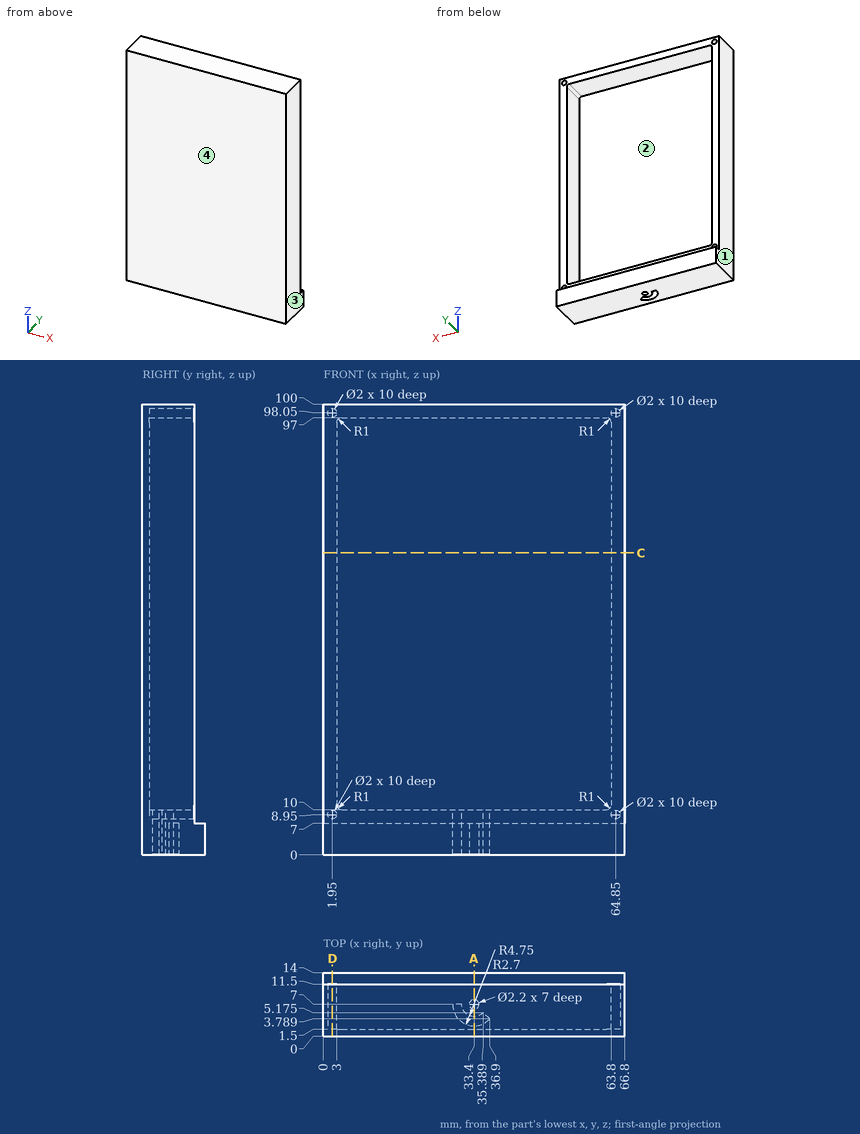
The figure shows three views and two pictorial views of one solid part (mm, origin at its lowest corner). Answer the questions. Give positions to 0.01 mm unless a question says otherwise; leave off trailing zeros. Order: outer loops, then holes, each group sorted by start corner. A loop starts at its lowest first (then second) coordinate and runs counter-clockwise, first axis right, second up. Notation, with made-up numbers: (-29.5, 49.5) -> (-9.5, 49.5) arc R9 cw to (-9.5, 63.5) -> close; hole circle Ø5 at (-16.5, 7.5). An arc over 180 degrees is marked (long way). Answer as CSV lines item,"result". Start each with the question number.
Q1. Determine the mould class of the marked faces 1, 2, 3 and 4 for opening direction X: pulls with the +X half, pulls with the -X half, needs draft (parallel to the pull), parting line crosses it, or undercut.
Q2. Given pin 1 (2 mm diameter, centred on x = 65, z = 9, fed in from +Y), flat-ended and moving along its own axis, determine where the tip first touches the part or whether it passes through.
Q3. A cutting plane is placed at C-C (z = 67). Determine the outline of the cut face in (x, y).
Q4. A cutting plane is placed at D-D (x = 1.95). Determine the outline of the cut face in (y, z).
Q5. A cutting plane is placed at A-A (x = 33.4). Determine the outline of the cut face in (y, z).
Q6. Find the intervals of material crossed by L1, parallel to Y at x = 33.4, z = 2; L2, parallel to X at y = 6.25, z = 50; L3, parallel to Z at x = 6.5, y = 10.25, in increasing order.
Results found:
1,face 1,"pulls with the -X half"
1,face 2,"undercut"
1,face 3,"pulls with the +X half"
1,face 4,"needs draft"
2,pin 1,"y = 11.5"
3,outline,"(0, 0) -> (66.8, 0) -> (66.8, 11.5) -> (63.8, 11.5) -> (63.8, 1.5) -> (3, 1.5) -> (3, 11.5) -> (0, 11.5) -> close"
4,outline,"(0, 0) -> (14, 0) -> (14, 7) -> (11.5, 7) -> (11.5, 7.95) -> (1.5, 7.95) -> (1.5, 9.95) -> (11.5, 9.95) -> (11.5, 97.05) -> (1.5, 97.05) -> (1.5, 99.05) -> (11.5, 99.05) -> (11.5, 100) -> (0, 100) -> close"
5,outline,"(0, 0) -> (2.25, 0) -> (2.25, 10) -> (1.5, 10) -> (1.5, 97) -> (11.5, 97) -> (11.5, 100) -> (0, 100) -> close; (4.3, 0) -> (5.9, 0) -> (5.9, 7) -> (8.1, 7) -> (8.1, 0) -> (14, 0) -> (14, 7) -> (11.5, 7) -> (11.5, 10) -> (4.3, 10) -> close"
6,L1,"0 to 2.25, 4.3 to 5.9, 8.1 to 14"
6,L2,"0 to 3, 63.8 to 66.8"
6,L3,"0 to 10, 97 to 100"
